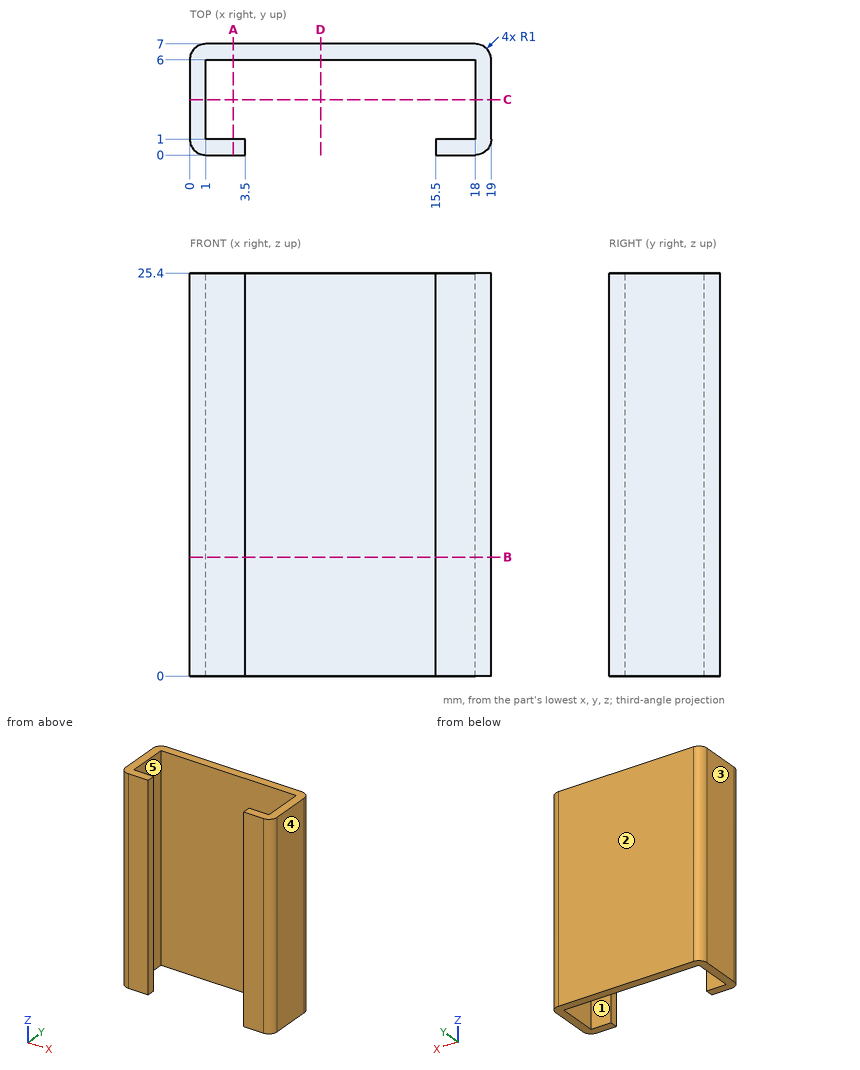
The drawing under review shows one solid part. Ordinate dimensions are in mm from its lowest x, y, z. A direction names the side the tool comes from. Give positions to 0.01 mm unless a question says otherwise; leave off trailing zeros. Order: outer loops, then holes, each group sorted by start corner. A loop starts at its lowest first (then second) coordinate and runs counter-clockwise, first axis right, second up. Notation, with made-up numbers: (-5, 35.25) -> (52, 35.25) arc R35 ccw to (52, 68.25) -> close; hole circle Ø2 at (-18, -18). An arc over 180 degrees is marked (long way). Write item = value, one per line.
1) Draft analysis for pull direction X (two halves, no side actions). For the marked faces 1, 2 and 3, state which applies: pulls with the +X half, pulls with the -X half, needs draft (parallel to the pull), parting line crosses it, or undercut.
Findings:
face_1 = undercut
face_2 = needs draft
face_3 = pulls with the -X half
2) Insertion check: pin 1 (0.5 mm diameter, centred on y = 0.5, z = 9.5, fed in from +X); pin 2 (8.5 mm diameter, centred on x = 10.5, z = 11, fed in from -Y). Each pin has a flat end and moves straight along its axis. Give the tip position at first contact, or say it passes through.
Findings:
pin_1 = 18.97
pin_2 = 6
3) We need section A-A, the plane x = 2.75. Give the boundary of the cut face in (y, z), and give its area (3 significant figures).
Findings:
outline = (0, 0) -> (1, 0) -> (1, 25.4) -> (0, 25.4) -> close; (6, 0) -> (7, 0) -> (7, 25.4) -> (6, 25.4) -> close
area = 50.8 mm^2
4) We need section B-B, the plane z = 7.5. Give the boundary of the cut face in (x, y), and give its area (3 significant figures).
Findings:
outline = (0, 1) arc R1 ccw to (1, 0) -> (3.5, 0) -> (3.5, 1) -> (1, 1) -> (1, 6) -> (18, 6) -> (18, 1) -> (15.5, 1) -> (15.5, 0) -> (18, 0) arc R1 ccw to (19, 1) -> (19, 6) arc R1 ccw to (18, 7) -> (1, 7) arc R1 ccw to (0, 6) -> close
area = 35.1 mm^2
5) We need section D-D, the plane x = 8.25. Give the boundary of the cut face in (y, z), and give its area (3 significant figures).
Findings:
outline = (6, 0) -> (7, 0) -> (7, 25.4) -> (6, 25.4) -> close
area = 25.4 mm^2
6) To check wall thickness, follow L1, parallel to X at y = 3, z = 14.25; L2, parallel to Y at x = 3.25, z = 20; L3, parallel to Y at x = 13.5, z = 11.5. State the ranges of each line that lie inside material, in increasing order. Write a range as from..to.
Findings:
L1 = 0..1, 18..19
L2 = 0..1, 6..7
L3 = 6..7
7) For the marked faces 4 and 5, list the 3-axis set-ups (+Z, -Z, +X, -X, +Y, -Y) from which the entire face can be reached by the end or side of a thin tool; tool diameter is ignored.
Findings:
face_4 = +Z, -Z, +X, +Y, -Y
face_5 = +Z, -Z
8) We need section C-C, the plane y = 3.5. Give the boundary of the cut face in (x, z).
Findings:
outline = (0, 0) -> (1, 0) -> (1, 25.4) -> (0, 25.4) -> close; (18, 0) -> (19, 0) -> (19, 25.4) -> (18, 25.4) -> close
